Input: part model. Units: mm. Frame: model coordinates. Face numbers are marked on the shaded views. A direction names the side the tool comes from. Round coordinates to 2 decimals unless told otherwise and drop trailing zeros. Loops run counter-clockwise (first coordinate to the right, second up) from the corner with the lowest first, then second, coordinate; pieces in that order, holes last. Notation, with made-up numbers: (74.25, 64.5) -> (104.25, 64.5) arc R29 cw to (104.25, 84.5) -> close; hole circle Ø1 at (84.25, -26.5). An arc over 180 degrees is marked (long way). Answer as a JSON object with one key per item and string values. Group by question number.
Item 1: Pin query (flat end, axial travel): pin 1 (15.5 mm diameter, centred on x = -1.5, y = 82, fed in from +Z); pin 2 (1.5 mm diameter, centred on x = -11, z = 10, fed in from +Y); pin 3 (20 mm diameter, centred on x = -4.5, y = 13, fed in from +Z). Return the tip coordinate at first contact, or that it passes through.
Item 2: Section query D-D on y = 0. Return loops of the section in (x, z), and give its area (3 significant figures).
Item 3: Material intervals for line 1 (X direction, y = -3, z = 24.5); line 2 (Z direction, x = -18, y = 30); line 3 (Y direction, x = -44, z = 31.5), sorted ascending. Write a range as [from, to].
Item 4: Section query C-C on x = 0. Return loops of the section in (y, z), and give its area (3 significant figures).
Item 5: Section query A-A on z = 35. Return loops of the section in (x, y).
Item 6: Set-up query: the marked faces 4, 5 and 6. Return all of +Z, -Z, +X, -X, +Y, -Y with unobstructed straight access to the full face (end or side cutting, diameter ignored); none if empty.
Item 7: Section query B-B on y = 49. Return loops of the section in (x, z).
Item 8: Draft query along Y for the marked faces 1, 2 and 3. Return one class per face: released by +Y, released by -Y, zero draft, split by the parting line, or undercut.
from build123d import *

# Parameters (mm, degrees)
BOSS_EXTRUDE1_DEPTH = 20
BOSS_EXTRUDE2_DEPTH = 30
CUT_EXTRUDE1_DEPTH  = 1
SKETCH8_R           = 15
CUT_EXTRUDE2_DEPTH  = 6
SKETCH9_R           = 11
CUT_EXTRUDE3_DEPTH  = 15
SKETCH10_R          = 7
CUT_EXTRUDE4_DEPTH  = 101


with BuildPart() as part:
    # Sketch3 → Boss-Extrude1 (new body)
    with BuildSketch(Plane.XY):
        with BuildLine():
            Line((-50, 103.561575886), (-50, -15.561575886))
            ThreePointArc((-50, -15.561575886), (0, -27), (50, -15.561575886))
            Line((50, -15.561575886), (50, 103.561575886))
            ThreePointArc((50, 103.561575886), (0, 115), (-50, 103.561575886))
        make_face()
        with BuildLine():
            ThreePointArc((30.545454545, 91.010852136), (0, 96), (-30.545454545, 91.010852136))
            ThreePointArc((-30.545454545, 91.010852136), (-35.584237678, 80.881159913), (-25.454545455, 75.84237678))
            ThreePointArc((-25.454545455, 75.84237678), (0, 80), (25.454545455, 75.84237678))
            ThreePointArc((25.454545455, 75.84237678), (35.584237678, 80.881159913), (30.545454545, 91.010852136))
        make_face(mode=Mode.SUBTRACT)
    extrude(amount=BOSS_EXTRUDE1_DEPTH)

    # Sketch5 → Boss-Extrude2 (add)
    with BuildSketch(Plane.XY.offset(20)):
        with BuildLine():
            Line((-50, 63), (-33, 63))
            Line((-33, 63), (-33, -22.163514831))
            ThreePointArc((-33, -22.163514831), (-41.631074926, -19.200063435), (-50, -15.561575886))
            Line((-50, -15.561575886), (-50, 63))
        make_face()
        with BuildLine():
            Line((50, -15.561575886), (50, 63))
            Line((50, 63), (33, 63))
            Line((33, 63), (33, -22.163514831))
            ThreePointArc((33, -22.163514831), (41.631074926, -19.200063435), (50, -15.561575886))
        make_face()
    extrude(amount=BOSS_EXTRUDE2_DEPTH)

    # Sketch6 → Cut-Extrude1 (cut)
    with BuildSketch(Plane.XY.offset(20)):
        with BuildLine():
            Line((-33, 63), (33, 63))
            Line((33, 63), (50, 63))
            Line((50, 63), (50, 103.561575886))
            ThreePointArc((50, 103.561575886), (0, 115), (-50, 103.561575886))
            Line((-50, 103.561575886), (-50, 63))
            Line((-50, 63), (-33, 63))
        make_face()
    extrude(amount=-CUT_EXTRUDE1_DEPTH, mode=Mode.SUBTRACT)

    # Sketch8 → Cut-Extrude2 (cut)
    with BuildSketch(Plane.XY.offset(20)):
        Circle(SKETCH8_R)
    extrude(amount=-CUT_EXTRUDE2_DEPTH, mode=Mode.SUBTRACT)

    # Sketch9 → Cut-Extrude3 (cut, through all)
    with BuildSketch(Plane.XY.offset(14)):
        Circle(SKETCH9_R)
    extrude(amount=-CUT_EXTRUDE3_DEPTH, mode=Mode.SUBTRACT)

    # Sketch10 → Cut-Extrude4 (cut, through all)
    with BuildSketch(Plane(origin=(50, 0, 0), x_dir=(0, 0, -1), z_dir=(1, 0, 0))):
        with Locations((-35, 49)):
            Circle(SKETCH10_R)
    extrude(amount=-CUT_EXTRUDE4_DEPTH, mode=Mode.SUBTRACT)


solid = part.part
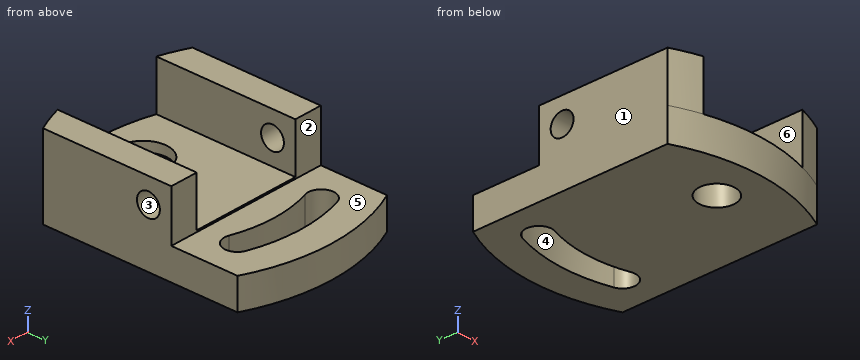
Solved:
{
 "1": {"pin 1": "z = 19", "pin 2": "y = 114.54", "pin 3": "z = 20"},
 "2": {"outline": "(-50, 0) -> (-11, 0) -> (-11, 14) -> (-15, 14) -> (-15, 20) -> (-33, 20) -> (-33, 50) -> (-50, 50) -> close; (11, 0) -> (50, 0) -> (50, 50) -> (33, 50) -> (33, 20) -> (15, 20) -> (15, 14) -> (11, 14) -> close", "area": "2,530 mm²"},
 "3": {"line 1": "[-50, -33], [33, 50]", "line 2": "[0, 20]", "line 3": "[-18.25, 42.94], [55.06, 63]"},
 "4": {"outline": "(-27, 0) -> (-11, 0) -> (-11, 14) -> (-15, 14) -> (-15, 20) -> (-27, 20) -> close; (11, 0) -> (80, 0) -> (80, 19) -> (63, 19) -> (63, 20) -> (15, 20) -> (15, 14) -> (11, 14) -> close; (96, 0) -> (115, 0) -> (115, 19) -> (96, 19) -> close", "area": "2,000 mm²"},
 "5": {"outline": "(-50, -15.56) arc R115 ccw to (-33, -22.16) -> (-33, 42) -> (-50, 42) -> close; (-50, 56) -> (-33, 56) -> (-33, 63) -> (-50, 63) -> close; (33, -22.16) arc R115 ccw to (50, -15.56) -> (50, 42) -> (33, 42) -> close; (33, 56) -> (50, 56) -> (50, 63) -> (33, 63) -> close"},
 "6": {"face 4": "+Z, -Z", "face 5": "+Z, +X, -X, +Y", "face 6": "+Z, +Y, -Y"},
 "7": {"outline": "(-50, 0) -> (50, 0) -> (50, 28) -> (33, 28) -> (33, 20) -> (-33, 20) -> (-33, 28) -> (-50, 28) -> close; (-50, 42) -> (-33, 42) -> (-33, 50) -> (-50, 50) -> close; (33, 42) -> (50, 42) -> (50, 50) -> (33, 50) -> close"},
 "8": {"face 1": "zero draft", "face 2": "released by +Y", "face 3": "undercut"}
}
